from build123d import *

# Parameters (mm, degrees)
CUT_EXTRUDE1_DEPTH = 9.525
CHAMFER1_SIZE      = 0.254
FILLET1_R          = 0.254


with BuildPart() as part:
    # Sketch1 → Revolve1 (revolve)
    with BuildSketch(Plane.XY):
        Polygon((0, 9.1694), (9.525, 9.1694), (9.525, 9.525), (11.43, 9.525), (11.43, 7.8867), (13.97, 7.8867), (13.97, 6.5), (39.37, 6.5), (39.37, 4.7625), (59.69, 4.7625), (59.69, 0), (0.635, 0), (0, 1.099852263), align=None)
    revolve(axis=Axis((0, 0, 0), (1, 0, 0)))

    # Sketch2 → Cut-Extrude1 (cut)
    with BuildSketch(Plane.ZY):
        with BuildLine():
            Line((-7.1501, -5.740554533), (-7.1501, 5.740554533))
            ThreePointArc((-7.1501, 5.740554533), (-9.1694, 0), (-7.1501, -5.740554533))
        make_face()
        with BuildLine():
            Line((7.1501, -5.740554533), (7.1501, 5.740554533))
            ThreePointArc((7.1501, 5.740554533), (9.1694, 0), (7.1501, -5.740554533))
        make_face()
    extrude(amount=-CUT_EXTRUDE1_DEPTH, mode=Mode.SUBTRACT)

    # Chamfer1
    chamfer1_edges = [part.edges().sort_by_distance(p)[0] for p in [
        (0, 9.1694, 0),
        (39.37, -6.5, 0),
        (0, 0, 7.1501),
        (0, -9.1694, 0),
        (0, 0, -7.1501),
        (59.69, -4.7625, 0),
    ]]
    chamfer(chamfer1_edges, length=CHAMFER1_SIZE)

    # Fillet1
    fillet1_edges = [part.edges().sort_by_distance(p)[0] for p in [
        (9.525, 9.1694, 0),
        (11.43, -7.8867, 0),
        (13.97, -6.5, 0),
        (9.525, 0, 7.1501),
        (9.525, -9.1694, 0),
        (9.525, 0, -7.1501),
        (39.37, -4.7625, 0),
    ]]
    fillet(fillet1_edges, radius=FILLET1_R)


solid = part.part
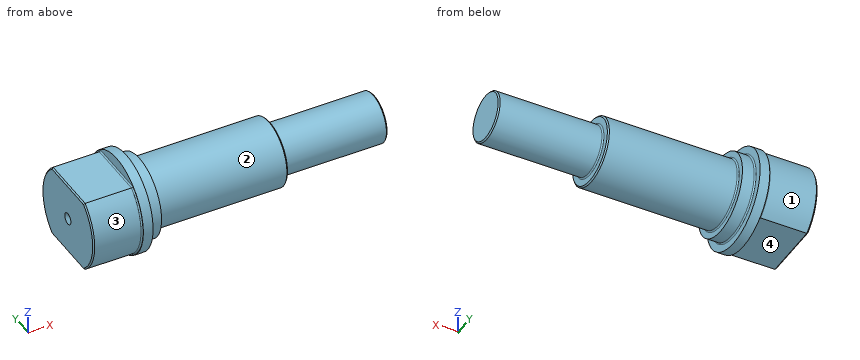
Part model, mm, in its own coordinate system. Face numbers are marked on the shaded views. A direction names the side the tool comes from. Coordinates: 2 decimals unless noted, no trailing zeros. Loops run counter-clockwise (first coordinate to the right, second up) from the corner with the lowest first, then second, coordinate; pieces in that order, holes last. Notation, with made-up numbers: (27.25, -1) -> (49.25, -1) arc R21 ccw to (49.25, 8) -> close; hole circle Ø10 at (86.25, 18). An arc over 180 degrees is marked (long way). Use a Markdown table: item, result. Add a question column.
Item 1: Band-saw the part on C-C on x = 50.5. Write the cut outline in (y, z) (1 decimal).
Item 2: Flat gauge pins, fed straight in: P1, Ø1, axis at y = 4.5, z = 4.5, coming from the +X side; P2, Ø5, axis at x = 35, z = 3.5, coming from the +Y side; P3, Ø2.5, axis at x = 5, y = 1.5, coming from the -Z side. Where does each tip first touch, or does it go through?
Item 3: Probe probe 1 along X at (y, z) = (0, 5.5); probe 2 along X at (y, z) = (-7.75, 5); probe 3 along Y at (x, z) = (53.5, -1.5). List the from-to ranges inside material, lowest first.
Item 4: Band-saw the part on A-A on x = 23. Write the cut outline in (y, z), plus the area to 3 significant figures.
Item 5: Band-saw the part on B-B on x = 8.5. Write the cut outline in (y, z).
Item 6: Which spindle directions (+Z, -Z, +X, -X, +Y, -Y) get a long thin tool onto all of the face, cutting with end or side? Do the marked faces 1, 2, 3 and 4. Say none if no direction does.
Geometry says:
| question | item | result |
|---|---|---|
| 1 | outline | circle Ø9.5 at (0, 0) |
| 2 | P1 | x = 39.37 |
| 2 | P2 | y = 6.42 |
| 2 | P3 | z = -7.15 |
| 3 | probe 1 | 0 to 39.37 |
| 3 | probe 2 | 9.43 to 11.43 |
| 3 | probe 3 | -4.52 to 4.52 |
| 4 | outline | circle Ø13 at (0, 0) |
| 4 | area | 133 mm² |
| 5 | outline | (-5.74, -7.15) -> (5.74, -7.15) arc R9.17 ccw to (5.74, 7.15) -> (-5.74, 7.15) arc R9.17 ccw to start |
| 6 | face 1 | -X, +Y |
| 6 | face 2 | +X |
| 6 | face 3 | -X, -Y |
| 6 | face 4 | -Z, -X, +Y, -Y |
